Autodesk Fusion 360 part; units mm, degrees
sketch "Sketch1" plane through (0, 0, 0) normal (0, 1, 0) x (1, 0, 0)
  line L0 (0, -11) -> (0, 10) construction
  line L1 (-3.875, 5.4644) -> (-3.875, 0.9922)
  line L2 (3.875, 0.9922) -> (3.875, 5.4644)
  arc A0 (-4.6875, 5.8547) -> (4.6875, 5.8547) centre (0, 0) ccw
  arc A1 (-3.875, 0.9922) -> (3.875, 0.9922) centre (0, 0) ccw
  arc A2 (-3.875, 5.4644) -> (-4.6875, 5.8547) centre (-4.375, 5.4644) ccw
  arc A3 (4.6875, 5.8547) -> (3.875, 5.4644) centre (4.375, 5.4644) ccw
  dimension "d1" = 8
  dimension "d2" = 15
  dimension "d4" = 0.5
  dimension "d5" = 7.75
extrude "Extrude1" add sketch "Sketch1" along normal blind 45.5
Geometry check sheet. Reference: the model listing, model coordinates, mm. A direction names the side the tool comes from. Coordinates: 2 decimals unless noted, no trailing zeros. Order: outer loops, then holes, each group sorted by start corner. A loop starts at its lowest first (then second) coordinate and runs counter-clockwise, first axis right, second up. Notation, with made-up numbers: M 50,87 L 87,87 A32 cw 87,126 Z; hole C 81,1 d5. An arc over 180 degrees is marked long. Answer as a JSON object with one key per item and string values.
Q1. Release check for a two-part mould opening along X. For faces 1 (the cylindrical face through (0.259, 22.432, 7.496)), 2 (the flat face through (-2, 0, 4)), 3 (the flat face through (-3.875, 22, -3)), 4 (the cylindrical face through (-4.17, 22.43, -5.92)) record: released by +X, released by -X, zero draft, split by the parting line, or undercut.
Results are:
{"face 1": "split by the parting line", "face 2": "zero draft", "face 3": "undercut", "face 4": "undercut"}
Q2. Cross-section at C-C on x = 0. Record the cut outline in (y, z).
Results are:
{"outline": "M 0,4 L 45.5,4 L 45.5,7.5 L 0,7.5 Z"}
Q3. Tool access check on faces 5 (the flat face through (3.875, 22, -3)), 6 (the cylindrical face through (0, 22, 4)). Record the directions out of +Z, -Z, +X, -X, +Y, -Y that give a thin tool (end or side, any length) a straight path to the whole face; none if there is none.
Results are:
{"face 5": "-Z, +Y, -Y", "face 6": "+Y, -Y"}
Q4. Depth check by flat-ended pin: pin 1 Ø2 at (y, z) = (18, -4) entering from +X; pin 2 Ø8 at (y, z) = (33, -1.5) entering from +X; pin 3 Ø5 at (x, z) = (0, 0) entering from -Y; pin 4 Ø1.5 at (y, z) = (41, 3.5) entering from -X. Enter the tip coordinate at first touch or a pass-through.
Results are:
{"pin 1": "stops at x = 6.87", "pin 2": "stops at x = 7.5", "pin 3": "passes through", "pin 4": "stops at x = -6.98"}
Q5. Cross-section at D-D on z = -3.5. Record the cut outline in (x, y) (3 decimals).
Results are:
{"outline": "M -6.633,0 L -3.875,0 L -3.875,45.5 L -6.633,45.5 Z; M 3.875,0 L 6.633,0 L 6.633,45.5 L 3.875,45.5 Z"}
Q6. Scan lines: line 1 (X direction, y = 10, z = 0); line 2 (Z direction, x = 0, y = 14.5); line 3 (X direction, y = 40, z = 0.75). Record each from-to range of solid material in increasing order.
Results are:
{"line 1": "x = -7.5 to -4, 4 to 7.5", "line 2": "z = 4 to 7.5", "line 3": "x = -7.46 to -3.93, 3.93 to 7.46"}
Q7. Cross-section at A-A on z = 0. Record the cut outline in (x, y).
Results are:
{"outline": "M -7.5,0 L -4,0 L -4,45.5 L -7.5,45.5 Z; M 4,0 L 7.5,0 L 7.5,45.5 L 4,45.5 Z"}
Q8. Cross-section at B-B on y = 10.5. Record the cut outline in (x, z) (1 decimal), and give its area (3 significant figures).
Results are:
{"outline": "M -4.7,-5.9 A0.5 ccw -3.9,-5.5 L -3.9,-1 A4 cw long 3.9,-1 L 3.9,-5.5 A0.5 ccw 4.7,-5.9 A7.5 ccw long Z", "area": "95.6 mm²"}
